Read the model definition and answer for the solid it produces. Units are mm, in the model's axes. A direction names the side the tool comes from. Give positions to 0.01 mm unless a question says otherwise; leave off trailing zeros. Loops run counter-clockwise (first coordinate to the right, second up) from the corner with the lowest first, then second, coordinate; pieces in that order, holes last. Notation, with made-up numbers: (-9, -19.5) -> (32, -19.5) arc R19 cw to (32, 8.5) -> close; hole circle Ø1 at (-23.5, 83.5). An arc over 180 degrees is marked (long way). One line per item, written item: value. Start each with the question number.
from build123d import *

# Parameters (mm, degrees)
SKETCH1_W             = 25.4
SKETCH1_H             = 25.4
SKETCH1_W_2           = 19.812
SKETCH1_H_2           = 19.812
BOSS_EXTRUDE1_DEPTH   = 33.02
SKETCH9_W             = 25.4
SKETCH9_H             = 25.4
BOSS_EXTRUDE5_DEPTH   = 12.7
SKETCH14_W            = 19.812
SKETCH14_H            = 19.812
SKETCH14_W_2          = 16.002
SKETCH14_H_2          = 16.002
BOSS_EXTRUDE6_DEPTH   = 2.54
SKETCH10_R            = 11
CUT_EXTRUDE1_DEPTH    = 7
CUT_EXTRUDE2_REACH    = 50.572
SKETCH15_R            = 5
SKETCH17_W            = 25.4
SKETCH17_H            = 25.4
BOSS_EXTRUDE7_DEPTH   = 6.35
CUT_EXTRUDE4_REACH    = 65.194
SKETCH18_R            = 6.5
CIRPATTERN1_COUNT     = 4
SKETCH23_R            = 3.2500062
CUT_EXTRUDE5_DEPTH    = 2.75
CIRPATTERN2_COUNT     = 4
FILLET3_R             = 12.7
FILLET4_R             = 1.27
FILLET5_R             = 1.27
F_4_CLEARANCE_HOLE1_D = 3.2639
CHAMFER1_SIZE         = 1.27


with BuildPart() as part:
    # Sketch1 → Boss-Extrude1 (new body)
    with BuildSketch(Plane(origin=(0, 0, 0), x_dir=(1, 0, 0), z_dir=(0, 1, 0))):
        Rectangle(SKETCH1_W, SKETCH1_H)
        Rectangle(SKETCH1_W_2, SKETCH1_H_2, mode=Mode.SUBTRACT)
    extrude(amount=BOSS_EXTRUDE1_DEPTH)

    # Sketch9 → Boss-Extrude5 (add)
    with BuildSketch(Plane.XZ):
        with Locations((-25.4, 0)):
            Rectangle(SKETCH9_W, SKETCH9_H)
    extrude(amount=-BOSS_EXTRUDE5_DEPTH)

    # Sketch14 → Boss-Extrude6 (add)
    with BuildSketch(Plane.XZ):
        Rectangle(SKETCH14_W, SKETCH14_H)
        Rectangle(SKETCH14_W_2, SKETCH14_H_2, mode=Mode.SUBTRACT)
    extrude(amount=-BOSS_EXTRUDE6_DEPTH)

    # Sketch10 → Cut-Extrude1 (cut)
    with BuildSketch(Plane(origin=(0, 12.7, 0), x_dir=(1, 0, 0), z_dir=(0, 1, 0))):
        with Locations(Location((-25.4, 0, 0), (0, 0, 270))):
            Circle(SKETCH10_R)
    extrude(amount=-CUT_EXTRUDE1_DEPTH, mode=Mode.SUBTRACT)

    # Sketch15 → Cut-Extrude2 (cut, up to next)
    with BuildSketch(Plane(origin=(0, 5.7, 0), x_dir=(1, 0, 0), z_dir=(0, 1, 0)), mode=Mode.PRIVATE) as cut_extrude2_sk1:
        with Locations(Location((-25.4, 0, 0), (0, 0, 270))):
            Circle(SKETCH15_R)
    cut_extrude2_tool1 = extrude(cut_extrude2_sk1.sketch, amount=-CUT_EXTRUDE2_REACH, mode=Mode.PRIVATE) & part.part
    add(cut_extrude2_tool1.solids().sort_by_distance((-25.4, 5.7, 0))[0], mode=Mode.SUBTRACT)

    # Sketch17 → Boss-Extrude7 (add)
    with BuildSketch(Plane.XZ):
        with Locations((-25.4, -25.4)):
            Rectangle(SKETCH17_W, SKETCH17_H)
    extrude(amount=-BOSS_EXTRUDE7_DEPTH)

    # Sketch18 → Cut-Extrude4 (cut, up to next)
    with BuildSketch(Plane.XZ, mode=Mode.PRIVATE) as cut_extrude4_sk1:
        with Locations(Location((-25.4, -25.4, 0), (0, 0, 270))):
            Circle(SKETCH18_R)
    cut_extrude4_tool1 = extrude(cut_extrude4_sk1.sketch, amount=-CUT_EXTRUDE4_REACH, mode=Mode.PRIVATE) & part.part
    add(cut_extrude4_tool1.solids().sort_by_distance((-25.4, 0, -25.4))[0], mode=Mode.SUBTRACT)

    # Sketch22 → M3 Clearance Hole1 (revolve, cut)
    with BuildSketch(Plane(origin=(-16.4, 0, -25.4), x_dir=(0, 0, -1), z_dir=(1, 0, 0))):
        Polygon((0, 0), (0, 13.721463052), (1.7, 12.7), (1.7, 0), align=None)
    m3_clearance_hole1 = revolve(axis=Axis((-16.4, -6.35, -25.4), (0, 1, 0)), mode=Mode.SUBTRACT)

    # CirPattern1: M3 Clearance Hole1 ×4 about axis
    cirpattern1_axis = Axis((-25.4, 0, -25.4), (0, 1, 0))
    for i in range(1, CIRPATTERN1_COUNT):
        add(m3_clearance_hole1.rotate(cirpattern1_axis, i * 360 / CIRPATTERN1_COUNT), mode=Mode.SUBTRACT)

    # Sketch23 → Cut-Extrude5 (cut)
    with BuildSketch(Plane(origin=(0, 6.35, 0), x_dir=(1, 0, 0), z_dir=(0, 1, 0))):
        with Locations((-25.4, 34.4)):
            Circle(SKETCH23_R)
    cut_extrude5 = extrude(amount=-CUT_EXTRUDE5_DEPTH, mode=Mode.SUBTRACT)

    # CirPattern2: Cut-Extrude5 ×4 about axis
    cirpattern2_axis = Axis((-25.4, 0, -25.4), (0, 1, 0))
    for i in range(1, CIRPATTERN2_COUNT):
        add(cut_extrude5.rotate(cirpattern2_axis, i * 360 / CIRPATTERN2_COUNT), mode=Mode.SUBTRACT)

    # Fillet3
    fillet3_edges = [part.edges().sort_by_distance(p)[0] for p in [
        (-38.1, 3.175, -38.1),
        (-12.7, 3.175, -38.1),
        (-38.1, 6.35, 12.7),
    ]]
    fillet(fillet3_edges, radius=FILLET3_R - 0.0001)  # a hair under: the kernel refuses the full size

    # Fillet4
    fillet4_edges = [part.edges().sort_by_distance(p)[0] for p in [
        (-8.001, 1.27, 8.001),
        (8.001, 1.27, 8.001),
        (8.001, 1.27, -8.001),
        (-8.001, 1.27, -8.001),
    ]]
    fillet(fillet4_edges, radius=FILLET4_R)

    # Fillet5
    fillet5_edges = [part.edges().sort_by_distance(p)[0] for p in [
        (-7.629025612, 2.54, -7.629025612),
        (-8.001, 2.54, 0),
        (-7.629025612, 2.54, 7.629025612),
        (0, 2.54, 8.001),
        (7.629025612, 2.54, 7.629025612),
        (8.001, 2.54, 0),
        (7.629025612, 2.54, -7.629025612),
        (-7.629025612, 0, -7.629025612),
        (-8.001, 0, 0),
        (-7.629025612, 0, 7.629025612),
        (0, 0, 8.001),
        (7.629025612, 0, 7.629025612),
        (8.001, 0, 0),
        (7.629025612, 0, -7.629025612),
        (0, 2.54, -8.001),
        (0, 0, -8.001),
    ]]
    fillet(fillet5_edges, radius=FILLET5_R - 0.0001)  # a hair under: the kernel refuses the full size

    # #4 Clearance Hole1 (through all)
    with Locations(Plane.XY.offset(12.7)):
        with Locations((0, 6.35)):
            Hole(F_4_CLEARANCE_HOLE1_D / 2)

    # Chamfer1
    chamfer1_edges = [part.edges().sort_by_distance(p)[0] for p in [
        (9.906, 33.02, 0),
        (0, 33.02, -9.906),
        (-9.906, 33.02, 0),
        (0, 33.02, 9.906),
    ]]
    chamfer(chamfer1_edges, length=CHAMFER1_SIZE)


solid = part.part
Item 1: Determine the mould class of faces 1 (the cylindrical face through (0.354, 4.757, 11.283)), 2 (the flat face through (-0.156, 32.376, -10.532)), 3 (the cylindrical face through (-34.48, 3.22, -34.28)) for opening direction Z: pulls with the +Z half, pulls with the -Z half, needs draft (parallel to the pull), parting line crosses it, or undercut.
Item 2: For faces 4 (the cylindrical face through (0.094, 0.362, -8.383)), 5 (the cylindrical face through (-23.45, 3.13, -31.6)), 6 (the flat face through (-20, 6.35, -20)), 7 (the flat face through (-33, 3.6, -24)), 8 (the flat face through (-12.7, 23, 0)), determine the directions among +Z, -Z, +X, -X, +Y, -Y from which every point of the face is accessible in a straight line to the end or side of a thin tool.
Item 3: Flat-ended cylindrical pins translate along their axes: pin 1 (5.5 mm diameter, centred on x = -25.4, z = -34.4, fed in from +Y); pin 2 (1.8 mm diameter, centred on x = -16, z = -25, fed in from +Y); pin 3 (10 mm diameter, centred on x = -4.5, y = 17, fed in from -Z); pin 4 (5 mm diameter, centred on x = -33, z = -11, fed in from +Y). Find the tip coordinate at first contact, or state that the pin passes through.
Item 4: Section A-A, the plane x = 0 is taken. State how many separate pieces and enclosed holes the cut face has, plus the area to 3 significant figures.
Item 5: Section C-C, the plane z = -16.4 is taken. Determine the outline of the cut face in (x, y).
Item 6: Section D-D, the plane y = 29 is taken. Determine the outline of the cut face in (x, z), plus the area to 3 significant figures.
Item 7: Section B-B, the plane y = 11.5 is taken. Determine the outline of the cut face in (x, z).
Item 8: Consider L1, parallel to Z at x = 6.5, y = 21; L2, parallel to X at y = 7.5, z = 0; L3, parallel to X at y = 4.55, z = -16.4. Determine where each line is inside the solid, lowest interval first. Write a range as [from, to].
Computed values:
1. face 1: needs draft
1. face 2: undercut
1. face 3: pulls with the -Z half
2. face 4: -Y
2. face 5: +Y, -Y
2. face 6: -Z, +X, -X, +Y
2. face 7: +Y
2. face 8: +Z, -Z, -X, +Y
3. pin 1: y = 3.6
3. pin 2: through
3. pin 3: z = -12.7
3. pin 4: y = 12.7
4. separate pieces: 4
4. enclosed holes: 0
4. area: 173 mm²
5. outline: (-38.1, 0) -> (-27.1, 0) -> (-27.1, 3.6) -> (-28.65, 3.6) -> (-28.65, 6.35) -> (-38.1, 6.35) -> close; (-23.7, 0) -> (-12.7, 0) -> (-12.7, 6.35) -> (-22.15, 6.35) -> (-22.15, 3.6) -> (-23.7, 3.6) -> close
6. outline: (-12.7, -12.7) -> (12.7, -12.7) -> (12.7, 12.7) -> (-12.7, 12.7) -> close; hole (-9.91, -9.91) -> (9.91, -9.91) -> (9.91, 9.91) -> (-9.91, 9.91) -> close
6. area: 253 mm²
7. outline: (-38.1, -12.7) -> (12.7, -12.7) -> (12.7, 12.7) -> (-25.4, 12.7) arc R12.7 ccw to (-38.1, 0) -> close; hole circle Ø22 at (-25.4, 0); hole (-9.91, -9.91) -> (9.91, -9.91) -> (9.91, 9.91) -> (-9.91, 9.91) -> close
8. L1: [-12.7, -9.91], [9.91, 12.7]
8. L2: [-38.1, -36.4], [-14.4, -9.91], [9.91, 12.7]
8. L3: [-38.1, -28.65], [-22.15, -12.7]
